Source: CAD feature listing. Evaluate the final solid. Frame: model axes, mm. A direction names the side the tool comes from. Give positions to 0.01 mm unless a question says otherwise; leave off trailing zeros. Loops run counter-clockwise (first coordinate to the right, second up) from the corner with the lowest first, then second, coordinate; pieces in that order, holes last. Notation, with made-up numbers: (-29.75, -2) - (23.25, -2) arc R17 ccw to (23.25, 18) - close; hole circle Ø9 at (-29, 34.25). An arc over 180 degrees is marked (long way). Write each question's results on one line, items separated by ' | '. Start each with the question number.
(1) Cut plane A-A on x = 0. Return the cut outline in (y, z).
(2) Pull-direction query (Z, two-part tool) for faces 4 (the flat face through (13, 0, -5)), 5 (the cylindrical face through (0.06, 0.43, 80.45)), 6 (the flat face through (4, -4, 65)); classes: pulls with the +Z half, pulls with the -Z half, needs draft (parallel to the pull), parting line crosses it, or undercut.
(3) Reachability of faces 1 (the cylindrical face through (2.08, 3.99, 73.87)), 2 (the cylindrical face through (15.5, -0.1, -2.5)), 3 (the cylindrical face through (-4.336, 19.524, 24.65)) from +Z, -Z, +X, -X, +Y, -Y: full face, straight path, thin tool, end or side. Return the list, or none.
(4) Cut plane C-C on z = 80. Return the cut outline in (x, y).
(5) Cut plane B-B on x = -14. Return the cut outline in (y, z), then the cut area to 3 significant figures.
(6) Contact query for flat-ended pins moving along their axis: pin 1 (8 mm diameter, centred on y = 3, z = 65.5, fed in from -X); pin 2 (10 mm diameter, centred on y = -9.5, z = 27.5, fed in from -X); pin 3 (8 mm diameter, centred on x = -7, z = 21, fed in from -Y). Output: stop coordinate, or through.
(7) Cut plane D-D on z = 43.5. Return the cut outline in (x, y), then the cut area to 3 significant figures.
(8) Material intervals for line 1 along Y through (x, z) = (0, 80); line 2 along Z through (x, y) = (2, -1); line 3 along Z through (x, y) = (-3.5, -12.5), sorted ascending. Write a range as [from, to].
Autodesk Inventor part; units mm, degrees
ref_plane "YZ Plane" through (0, 0, 0) normal (1, 0, 0) x (0, 1, 0)
ref_plane "XZ Plane" through (0, 0, 0) normal (0, 1, 0) x (-1, 0, 0)
ref_plane "XY Plane" through (0, 0, 0) normal (0, 0, 1) x (1, 0, 0)
sketch "Sketch1" plane through (0, 0, 0) normal (0, 0, 1) x (1, 0, 0)
  circle A0 centre (0, 0) radius 20
  dimension "d0" = 40
extrude "Extrusion1" add sketch "Sketch1" along normal blind 50
sketch "Sketch2" plane through (0, 0, 50) normal (0, 0, 1) x (1, 0, 0)
  circle A0 centre (0, 0) radius 8.5
  dimension "d3" = 17
extrude "Extrusion2" add sketch "Sketch2" along normal blind 15
thread "Thread1"
sketch "Sketch3" plane through (0, 0, 65) normal (0, 0, 1) x (1, 0, 0)
  circle A0 centre (0, 0) radius 4.5
  dimension "d8" = 9
extrude "Extrusion3" add sketch "Sketch3" along normal blind 20
sketch "Sketch4" plane through (0, 0, 0) normal (1, 0, 0) x (0, 1, 0)
  line L0 (4.5, 85) -> (-4.5, 85)
  line L1 (0, 85) -> (0, 80)
  circle A0 centre (0, 80) radius 1
  circle A1 centre (-1, 80) radius 1.5
  point P0 (0, 0)
  dimension "d11" = 5
  dimension "d12" = 3
extrude "Extrusion4" cut sketch "Sketch4" along normal through all both and the other way through all contours A1 A0 L1 | L1 A0 A1 | A0 A1 picked at (0.0001, 79.7835)
fillet "Fillet1" radius 2 1 edges at (-4.5, 0, 85)
sketch "Sketch5" plane through (0, 0, 0) normal (0, 0, -1) x (-1, 0, 0)
  circle A0 centre (14, 0) radius 2.5
  circle A1 centre (-13, 0) radius 2.5
  point P0 (0, 0)
  dimension "d16" = 5
  dimension "d17" = 5
extrude "Extrusion5" add sketch "Sketch5" along normal blind 5
properties part number "dc motor for capping system"
Ans:
1) outline: (-20, 0) - (20, 0) - (20, 50) - (8.5, 50) - (8.5, 65) - (4.5, 65) - (4.5, 83) arc R2 ccw to (2.5, 85) - (-2.5, 85) arc R2 ccw to (-4.5, 83) - (-4.5, 65) - (-8.5, 65) - (-8.5, 50) - (-20, 50) - close; hole circle Ø3 at (-1, 80)
2) face 4: pulls with the -Z half | face 5: undercut | face 6: pulls with the +Z half
3) face 1: +Z | face 2: -Z | face 3: +Z, -Z
4) outline: (-4.47, 0.5) - (4.47, 0.5) arc R4.5 ccw to start; (-3.74, -2.5) arc R4.5 ccw to (3.74, -2.5) - close
5) outline: (-14.28, 0) - (-2.5, 0) - (-2.5, -5) - (2.5, -5) - (2.5, 0) - (14.28, 0) - (14.28, 50) - (-14.28, 50) - close | area: 1,450 mm^2
6) pin 1: x = -8.5 | pin 2: x = -19.49 | pin 3: y = -19.77
7) outline: circle Ø40 at (0, 0) | area: 1,260 mm^2
8) line 1: [-4.5, -2.5], [0.5, 4.5] | line 2: [0, 78.5], [81.5, 85] | line 3: [0, 50]
